from build123d import *

# Parameters (mm, degrees)
BASE_FLANGE1_DEPTH           = 3.2639
EDGE_FLANGE1_DEPTH           = 1016
EDGE_FLANGE2_DEPTH           = 1016
BOSS_EXTRUDE1_DEPTH          = 3.2639
CUT_EXTRUDE1_DEPTH           = 3.2639
F_10_0_1935_DIAMETER_HOLE1_D = 4.9149
LPATTERN1_COUNT              = 4
LPATTERN1_PITCH              = 155.575
F_3_8_0_4_DOWEL_HOLE1_D      = 10.16
F_10_0_1935_DIAMETER_HOLE2_D = 4.9149
F_10_0_1935_DIAMETER_HOLE3_D = 4.9149
FILLET1_R                    = 6.35


# Sheet-metal steps are written as plain solids
with BuildPart() as part:
    # Sketch1 → Base-Flange1 (new body)
    with BuildSketch(Plane.XY):
        Polygon((0, 0), (653.072211442, 778.301154209), (576.30897854, 778.301154209), (0, 91.482858589), align=None)
    extrude(amount=-BASE_FLANGE1_DEPTH)

    # Edge-Flange1 section (across the edge) → Edge-Flange1 (add)
    with BuildSketch(Plane(origin=(654.045087884, 777.484813945, -3.2639), x_dir=(-0.7660444431189772, 0.6427876096865405, -3.4914813388431334e-15), z_dir=(-0.6427876096865405, -0.7660444431189772, 0))):
        with BuildLine():
            Line((-3.2639, 1.27), (-3.2639, 68.58))
            Line((-3.2639, 68.58), (0, 68.58))
            Line((0, 68.58), (0, 1.27))
            ThreePointArc((0, 1.27), (0.371974388, 0.371974388), (1.27, 0))
            Line((1.27, 0), (1.27, -3.2639))
            ThreePointArc((1.27, -3.2639), (-1.935951435, -1.935951435), (-3.2639, 1.27))
        make_face()
    extrude(amount=EDGE_FLANGE1_DEPTH)

    # Edge-Flange2 section (across the edge) → Edge-Flange2 (add)
    with BuildSketch(Plane(origin=(654.045087884, 777.484813945, -73.1139), x_dir=(0, 0, 1), z_dir=(-0.6427876096865404, -0.7660444431189771, 0))):
        with BuildLine():
            Line((-3.2639, 1.27), (-3.2639, 9.4361))
            Line((-3.2639, 9.4361), (0, 9.4361))
            Line((0, 9.4361), (0, 1.27))
            ThreePointArc((0, 1.27), (0.371974388, 0.371974388), (1.27, 0))
            Line((1.27, 0), (1.27, -3.2639))
            ThreePointArc((1.27, -3.2639), (-1.935951435, -1.935951435), (-3.2639, 1.27))
        make_face()
    extrude(amount=EDGE_FLANGE2_DEPTH)

    # Sketch12 → Boss-Extrude1 (add)
    with BuildSketch(Plane(origin=(0, 0, -76.3778), x_dir=(-1, 0, 0), z_dir=(0, 0, -1))):
        Polygon((-576.30897854, 778.301154209), (-653.072211442, 778.301154209), (0, 0), (0, 91.482858589), align=None)
    extrude(amount=-BOSS_EXTRUDE1_DEPTH)

    # Sketch13 → Cut-Extrude1 (cut)
    with BuildSketch(Plane(origin=(0, 0, -76.3778), x_dir=(-1, 0, 0), z_dir=(0, 0, -1))):
        Polygon((-646.816615915, 783.550222108), (-653.072211442, 778.301154209), (-642.412124976, 778.301154209), align=None)
        Polygon((0, 12.704196343), (0, 0), (6.255595527, 5.249067899), align=None)
    extrude(amount=-CUT_EXTRUDE1_DEPTH, mode=Mode.SUBTRACT)

    # #10 (0.1935) Diameter Hole1 (through all)
    with Locations(Plane.XY):
        with Locations((456.639396233, 613.457095394)):
            f_10_0_1935_diameter_hole1 = Hole(F_10_0_1935_DIAMETER_HOLE1_D / 2)

    # LPattern1: #10 (0.1935) Diameter Hole1 ×4
    with Locations(*[Vector(-0.6427876096865404, -0.7660444431189771, 0) * (i * LPATTERN1_PITCH) for i in range(1, LPATTERN1_COUNT)]):
        add(f_10_0_1935_diameter_hole1, mode=Mode.SUBTRACT)

    # 3/8 (0.4) Dowel Hole1 (through all)
    with Locations(Plane.XY):
        with Locations((56.751746801, 136.647718392), (81.073657871, 116.239211785), (130.054073729, 174.611798351), (105.73216266, 195.020304958)):
            Hole(F_3_8_0_4_DOWEL_HOLE1_D / 2)

    # #10 (0.1935) Diameter Hole2 (through all)
    with Locations(Plane.XY):
        with Locations((12.7, 30.488995291), (22.225, 52.713995291), (22.225, 79.701495291), (22.225, 106.688995291)):
            Hole(F_10_0_1935_DIAMETER_HOLE2_D / 2)

    # #10 (0.1935) Diameter Hole3 (through all)
    with Locations(Plane.XY):
        with Locations((581.956041646, 765.273369352), (532.975625788, 706.900782786), (562.161919071, 682.410574857), (611.142334929, 740.783161423)):
            Hole(F_10_0_1935_DIAMETER_HOLE3_D / 2)

    # Fillet1
    fillet1_edges = [part.edges().sort_by_distance(p)[0] for p in [
        (0, 91.482858589, -74.74585),
        (576.30897854, 778.301154209, -74.74585),
        (0, 91.482858589, -1.63195),
        (576.30897854, 778.301154209, -1.63195),
    ]]
    fillet(fillet1_edges, radius=FILLET1_R)


solid = part.part
Design review of the part built by this model. Coordinates are the model's own, in mm. A direction names the side the tool comes from. Coordinates: 2 decimals unless noted, no trailing zeros. Loops run counter-clockwise (first coordinate to the right, second up) from the corner with the lowest first, then second, coordinate; pieces in that order, holes last. Notation, with made-up numbers: M -8.75,22.25 L -2.75,22.25 A33 ccw -2.75,61.25 Z; hole C 31,-2 d1. An arc over 180 degrees is marked long. Use one line per item in the form item = value.
(1) For line 1 along Z through (x, y) = (382, 495); line 2 along X through (y, z) = (738, -58); line 3 along X through (y, z) = (108, -16.5), list the stretches that pass through material, from the lowest coordinate up. Write a range as from..to.
Return value:
line_1 = -76.38..-73.11, -3.26..0
line_2 = 620.91..625.17
line_3 = 92.28..96.54
(2) Clearance check with flat-ended pins moving along their axes: P1, Ø3, axis at x = 532.98, y = 706.9, coming from the +Z side; P2, Ø5.5, axis at x = 562.16, y = 682.41, coming from the +Z side; P3, Ø3, axis at y = 317.5, z = -17.5, coming from the -X side; P4, Ø4, axis at x = 81, z = -24.5, coming from the -Y side. State where each tip first meets the part, or that it passes through.
Return value:
P1 = through
P2 = 0
P3 = 266.81
P4 = 87.1
(3) Draft analysis for pull direction Z (two halves, no side actions). For faces 1 (the face through (301, 391, -3.264)), 2 (the face through (304, 420, -76.378)), 3 (the face through (291.956, 439.423, -1.609)), 4 (the face through (304, 420, -73.114)), state which applies: pulls with the +Z half, pulls with the -Z half, needs draft (parallel to the pull), parting line crosses it, or undercut.
Return value:
face_1 = undercut
face_2 = pulls with the -Z half
face_3 = needs draft
face_4 = undercut
(4) Consider section A-A (z = -49). Write out the cut boundary in (x, y), and give its area (3 significant figures).
Return value:
outline = M 0.97,-0.82 L 3.47,-2.91 L 656.55,775.39 L 654.05,777.48 Z
area = 3,320 mm2
(5) For faces 5 (the face through (301, 391, 0)), 6 (the face through (331.803, 394.015, -3.646)), list the 3-axis set-ups (+Z, -Z, +X, -X, +Y, -Y) from which the entire face can be reached by the end or side of a thin tool; tool diameter is ignored.
Return value:
face_5 = +Z, +X, -X, +Y, -Y
face_6 = -X, +Y
